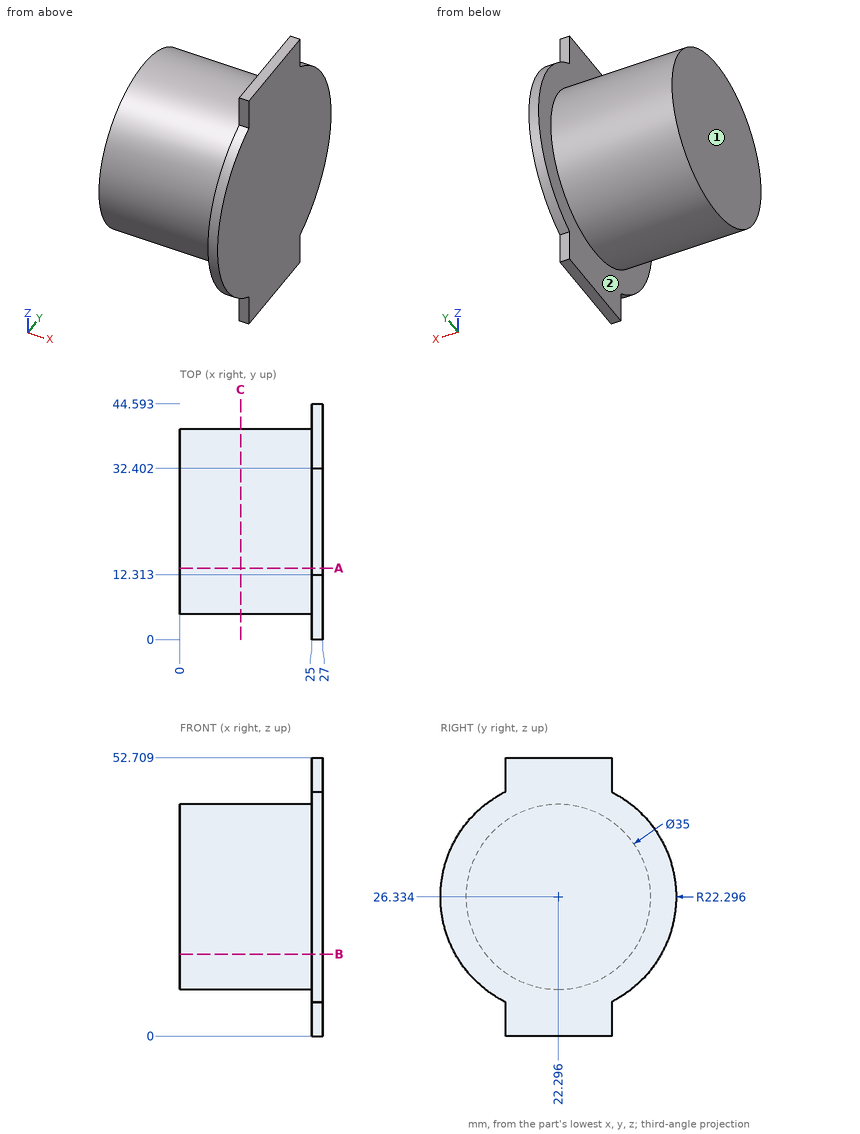
Print and shaded views of the part. All mm, measured from the part's lowest x, y and z. A direction names the side the tool comes from. Round coordinates to 2 decimals unless told otherwise and drop trailing zeros. Write each loop counter-clockwise with the first axis right and the second up, starting at its lowest first coordinate (ties: lowest second). Pieces come first, ordered by that corner, then holes. Notation, with made-up numbers: (55.5, 17) - (73.5, 17) arc R16 cw to (73.5, 33) - close; hole circle Ø10 at (-39.75, -23.75). An arc over 180 degrees is marked (long way). One line per item, written item: value.
(1) 3-axis set-ups, long thin cutter, end or side, ignore diameter. For the marked faces 1 and 2: which of +Z, -Z, +X, -X, +Y, -Y reach the whole face in a straight line?
Values follow:
face 1: +Z, -Z, -X, +Y, -Y
face 2: -X
(2) Cut at C-C, the plane x = 11.5. Give the cut face in (y, z) (1 decimal), plus the area to 3 significant figures.
Values follow:
outline: circle Ø35 at (22.3, 26.3)
area: 962 mm²
(3) Drop flat-ended pins along their axis: P1, Ø0.6, axis at x = 26, z = 2.5, coming from the -Y side; P2, Ø0.6, axis at x = 25.5, z = 4, coming from the +Y side; P3, Ø5, axis at y = 8, z = 43.5, coming from the -X side; P4, Ø5, axis at y = 28.5, z = 44, coming from the -X side. Give the stop position or say it passes through.
Values follow:
P1: stops at y = 12.31
P2: stops at y = 32.4
P3: stops at x = 25
P4: stops at x = 0
(4) Cut at A-A, the plane y = 13.5. Give the cut face in (x, z) (1 decimal), plus the area to 3 significant figures.
Values follow:
outline: (0, 11.2) - (25, 11.2) - (25, 0) - (27, 0) - (27, 52.7) - (25, 52.7) - (25, 41.5) - (0, 41.5) - close
area: 862 mm²
(5) Wall check: probe 1 along Y at (x, z) = (15.5, 27); probe 2 along X at (y, z) = (38.5, 17); probe 3 along Z at (x, y) = (15.25, 14) (1 decimal). Give the ranges that are in metal, low to high.
Values follow:
probe 1: y = 4.81 to 39.78
probe 2: x = 25 to 27
probe 3: z = 10.9 to 41.7
(6) Cut at B-B, the plane z = 15.5. Give the cut face in (x, y).
Values follow:
outline: (0, 8.55) - (25, 8.55) - (25, 2.81) - (27, 2.81) - (27, 41.78) - (25, 41.78) - (25, 36.04) - (0, 36.04) - close
